Geometry: final body of the model. Coordinates: model frame, mm. A direction names the side the tool comes from. Give positions to 0.01 mm unless a question says otherwise; leave off trailing zeros. Write each loop counter-clockwise with the first axis right and the second up, starting at its lowest first coordinate (ties: lowest second). Pieces come first, ordered by that corner, then holes. Notation, with made-up numbers: (48, 81) -> (107, 81) arc R20 ccw to (107, 103) -> close; hole circle Ø7 at (9.25, 12.5). An arc over 180 degrees is marked (long way). Answer in a Markdown table with one row per item. Add a question column.
Item 1: Section query D-D on z = 9.25. Output: boundary loops of the cut face in (x, y), plus the area to 3 significant figures.
Item 2: First-contact query: P1, Ø4, axis at x = 9, z = 0.5, coming from the -Y side; P2, Ø3, axis at x = 15, z = 6, coming from the +Y side; P3, Ø2, axis at x = 20, y = -2, coming from the -Z side; P4, Ø0.8, axis at x = 16, y = -3, coming from the -Z side. Flat tips, straight axial feed; report the tip coordinate or a pass-through.
Item 3: Section query C-C on y = 2.5. Output: boundary loops of the cut face in (x, z).
Item 4: Access query for faces 1 (the cylindrical face through (-1, -2, 0)), 2 (the cylindrical face through (36, -2, 0)), 3 (the cylindrical face through (43, 0, 10)). Directions: +Z, -Z, +X, -X, +Y, -Y. A direction counts if a zero-diameter tool reaches every point of the face in a straight line with its end or side. Return the directions, or none.
Item 5: Section query A-A on z = 7. Output: boundary loops of the cut face in (x, y), plus the area to 3 significant figures.
Item 6: Section query B-B on x = 25.5. Output: boundary loops of the cut face in (y, z), plus the area to 3 significant figures.
Item 7: Material intervals for probe 1 along X at (y, z) = (-2.6, 7); probe 2 along X at (y, z) = (-3, 6); probe 3 along Y at (x, z) = (21, 4.5), sorted ascending. Write a range as from..to.
```python
from build123d import *

# Parameters (mm, degrees)
SKETCH_6_R      = 3.5
EXTRUDE_4_DEPTH = 8
EXTRUDE_START   = -24
SKETCH_7_R      = 3.5
EXTRUDE_5_DEPTH = 8
EXTRUDE_START_2 = -3.5
SKETCH_8_R      = 1.5
EXTRUDE_6_DEPTH = 1.5
SKETCH_10_R     = 2


with BuildPart() as part:
    # Sketch 6 → Extrude 4 (new body)
    with BuildSketch(Plane(origin=(0, 0, 0), x_dir=(0, 0, -1), z_dir=(1, 0, 0))):
        Circle(SKETCH_6_R)
    extrude(amount=EXTRUDE_4_DEPTH)



with BuildPart() as body_2:
    # Sketch 7 → Extrude 5 (new body)
    with BuildSketch(Plane.ZY.offset(EXTRUDE_START)):
        with Locations(Location((0, 0, 0), (0, 0, 180))):
            Circle(SKETCH_7_R)
    extrude(amount=-EXTRUDE_5_DEPTH)


with BuildPart() as part_1:
    add(part.part)

    add(body_2.part)  # Extrude 6 merges body 2
    # Sketch 8 → Extrude 6 (add)
    with BuildSketch(Plane(origin=(0, 0, 0), x_dir=(1, 0, 0), z_dir=(0, 1, 0)).offset(EXTRUDE_START_2)):
        Polygon((0, 0), (8, 0), (8, -3.5), (24, -3.5), (24, 0), (32, 0), (32, -13.5), (0, -13.5), align=None)
        with Locations(Location((25.5, -7, 0), (0, 0, 270))):
            Circle(SKETCH_8_R, mode=Mode.SUBTRACT)
        with Locations(Location((6.5, -7, 0), (0, 0, 270))):
            Circle(SKETCH_8_R, mode=Mode.SUBTRACT)
    extrude(amount=EXTRUDE_6_DEPTH)

    # Sweep 1: sweep along a path in Sketch 9
    with BuildLine(Plane(origin=(0, 0, 0), x_dir=(1, 0, 0), z_dir=(0, 1, 0))) as sweep_1_path:
        Line((-5, 0), (39, 0))
        ThreePointArc((39, 0), (43.242640687, -1.757359313), (45, -6))
        Line((45, -6), (45, -13.5))
    # Sketch 10 → Sweep 1 (sweep)
    with BuildSketch(Plane(origin=(-5, 0, 0), x_dir=(0, 0, -1), z_dir=(1, 0, 0))):
        Circle(SKETCH_10_R)
    sweep(path=sweep_1_path.line)

    # Sketch 11 → Cut-Revolve 1 (revolve, cut)
    with BuildSketch(Plane(origin=(0, 0, 0), x_dir=(1, 0, 0), z_dir=(0, 1, 0))):
        Polygon((-2, 2), (-5, 2), (-5, 1.4), align=None)
    revolve(axis=Axis((-14.922922677, 0, 0), (1, 0, 0)), mode=Mode.SUBTRACT)


solid = part_1.part
```
Findings below:
| question | item | result |
|---|---|---|
| 1 | outline | (0, -3.5) -> (32, -3.5) -> (32, -2) -> (0, -2) -> close; circle Ø4 at (45, 0) |
| 1 | area | 60.6 mm^2 |
| 2 | P1 | stops at y = -3.5 |
| 2 | P2 | stops at y = -2 |
| 2 | P3 | stops at z = -1.73 |
| 2 | P4 | stops at z = 3.5 |
| 3 | outline | (0, -2.45) -> (8, -2.45) -> (8, 2.45) -> (0, 2.45) -> close; (24, -2.45) -> (32, -2.45) -> (32, 2.45) -> (24, 2.45) -> close |
| 4 | face 1 | -X |
| 4 | face 2 | none |
| 4 | face 3 | +Z |
| 5 | outline | (0, -3.5) -> (5, -3.5) -> (5, -2) -> (0, -2) -> close; (8, -3.5) -> (24, -3.5) -> (24, -2) -> (8, -2) -> close; (27, -3.5) -> (32, -3.5) -> (32, -2) -> (27, -2) -> close; circle Ø4 at (45, 0) |
| 5 | area | 51.6 mm^2 |
| 6 | outline | (-3.5, 0) arc R3.5 ccw (long way) to (-2, 2.87) -> (-2, 5.5) -> (-3.5, 5.5) -> close; (-3.5, 8.5) -> (-2, 8.5) -> (-2, 13.5) -> (-3.5, 13.5) -> close |
| 6 | area | 51.2 mm^2 |
| 7 | probe 1 | x = 0..5, 8..24, 27..32 |
| 7 | probe 2 | x = 0..5.38, 7.62..24.38, 26.62..32 |
| 7 | probe 3 | y = -3.5..-2 |
